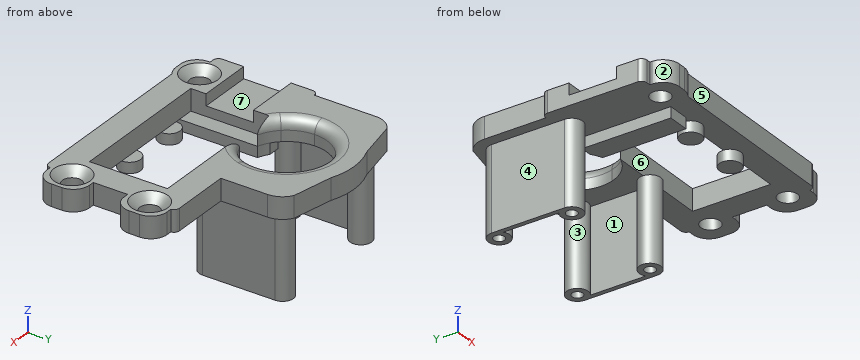
```python
from build123d import *

# Parameters (mm, degrees)
BOSS_EXTRUDE1_DEPTH                                  = 4
SKETCH5_W                                            = 5.2
SKETCH5_H                                            = 8.8
SKETCH5_W_2                                          = 5
CUT_EXTRUDE1_DEPTH                                   = 2.15
FILLET1_R                                            = 1
BOSS_EXTRUDE2_OUTLINE_R                              = 1
BOSS_EXTRUDE2_DEPTH                                  = 15.61
BOSS_EXTRUDE5_START                                  = -5
BOSS_EXTRUDE5_DEPTH                                  = 5
BOSS_EXTRUDE8_DEPTH                                  = 4
FILLET3_R                                            = 2
SKETCH9_R                                            = 2
BOSS_EXTRUDE9_DEPTH                                  = 2
SKETCH10_W                                           = 27.2
SKETCH10_H                                           = 14.5
SKETCH10_W_2                                         = 27
SKETCH10_H_2                                         = 14.3
CUT_EXTRUDE4_DEPTH                                   = 4
BOSS_EXTRUDE10_START                                 = 2
BOSS_EXTRUDE10_DEPTH                                 = 2
SKETCH12_W                                           = 8
SKETCH12_H                                           = 8
SKETCH12_W_2                                         = 6.2
SKETCH12_H_2                                         = 6.2
BOSS_EXTRUDE11_DEPTH                                 = 4
FILLET4_R                                            = 3
FILLET5_R                                            = 3
CSK_FOR_M3_HEX_SOCKET_COUNTERSUNK_CAP_SC_D           = 3.6
CSK_FOR_M3_HEX_SOCKET_COUNTERSUNK_CAP_SC_DEPTH       = 14.44
CSK_FOR_M3_HEX_SOCKET_COUNTERSUNK_CAP_SC_CSINK_D     = 6.72
CSK_FOR_M3_HEX_SOCKET_COUNTERSUNK_CAP_SC_CSINK_ANGLE = 90
CSK_FOR_M3_HEX_SOCKET_COUNTERSUNK_CAP_SC_TIP         = 1.081549114


# Read off the part's stored shape, not the designer's step: Boss-Extrude2
with BuildPart() as part:
    # Sketch3 → Boss-Extrude1 (new body)
    with BuildSketch(Plane.XY):
        with BuildLine():
            Line((5, 19.3), (-9.345122918, 19.3))
            ThreePointArc((-9.345122918, 19.3), (-23.0857932, 33.91726612), (-33.128131381, 16.55))
            Line((-33.128131381, 16.55), (-37.2, 16.55))
            Line((-37.2, 16.55), (-37.2, -2.25))
            Line((-37.2, -2.25), (-32, -2.25))
            Line((-32, -2.25), (-32, -5))
            Line((-32, -5), (5, -5))
            Line((5, -5), (5, 19.3))
        make_face()
        with BuildLine():
            ThreePointArc((-23.75, 14.3), (-25.677557149, 15.173169561), (-27.284491991, 16.55))
            ThreePointArc((-27.284491991, 16.55), (-19.55505766, 28.701473224), (-19.55, 14.3))
            Line((-19.55, 14.3), (0, 14.3))
            Line((0, 14.3), (0, 0))
            Line((0, 0), (-27, 0))
            Line((-27, 0), (-27, 14.3))
            Line((-27, 14.3), (-23.75, 14.3))
        make_face(mode=Mode.SUBTRACT)
    extrude(amount=BOSS_EXTRUDE1_DEPTH)

    # Sketch5 → Cut-Extrude1 (cut)
    with BuildSketch(Plane.XY.offset(4)):
        with Locations((-29.6, 7.15)):
            Rectangle(SKETCH5_W, SKETCH5_H)
        with Locations((-34.7, 7.15)):
            Rectangle(SKETCH5_W_2, SKETCH5_H)
    extrude(amount=-CUT_EXTRUDE1_DEPTH, mode=Mode.SUBTRACT)

    # Fillet1
    fillet1_edges = [part.edges().sort_by_distance(p)[0] for p in [
        (5, 19.3, 2),
        (5, -5, 2),
        (-32, -5, 2),
        (-32, -2.25, 2),
        (-37.2, -2.25, 2),
        (-37.2, 16.55, 2),
    ]]
    fillet(fillet1_edges, radius=FILLET1_R)

    # Boss-Extrude2 outline → Boss-Extrude2 (add)
    # profile 1 of 2: a face of its own
    with BuildSketch(Plane.XY.offset(-15.61)):
        with BuildLine():
            ThreePointArc((-9.15, 28), (-12.938854382, 28.894427191), (-9.95, 26.4))
            Line((-9.95, 26.4), (-9.95, 16.1))
            ThreePointArc((-9.95, 16.1), (-12.938854382, 13.605572809), (-9.15, 14.5))
            Line((-9.15, 14.5), (-9.15, 28))
        make_face()
        with Locations((-11.15, 14.5)):
            Circle(BOSS_EXTRUDE2_OUTLINE_R, mode=Mode.SUBTRACT)
        with Locations((-11.15, 28)):
            Circle(BOSS_EXTRUDE2_OUTLINE_R, mode=Mode.SUBTRACT)
    # profile 2 of 2: a face of its own
    with BuildSketch(Plane.XY.offset(-15.61)):
        with BuildLine():
            ThreePointArc((-33.35, 26.4), (-30.361145618, 28.894427191), (-34.15, 28))
            Line((-34.15, 28), (-34.15, 14.5))
            ThreePointArc((-34.15, 14.5), (-30.361145618, 13.605572809), (-33.35, 16.1))
            Line((-33.35, 16.1), (-33.35, 26.4))
        make_face()
        with Locations((-32.15, 14.5)):
            Circle(BOSS_EXTRUDE2_OUTLINE_R, mode=Mode.SUBTRACT)
        with Locations((-32.15, 28)):
            Circle(BOSS_EXTRUDE2_OUTLINE_R, mode=Mode.SUBTRACT)
    extrude(amount=BOSS_EXTRUDE2_DEPTH)

    # Sketch7 → Boss-Extrude5 (add)
    with BuildSketch(Plane.XY.offset(BOSS_EXTRUDE5_START)):
        with BuildLine():
            Line((-13.139974874, 14.3), (-11.15, 15.313011827))
            Line((-11.15, 15.313011827), (-9.160025126, 14.3))
            ThreePointArc((-9.160025126, 14.3), (-11.15, 12.5), (-13.139974874, 14.3))
        make_face()
    extrude(amount=BOSS_EXTRUDE5_DEPTH)

    # Sketch8 → Boss-Extrude8 (add)
    with BuildSketch(Plane(origin=(0, 0, 0), x_dir=(-1, 0, 0), z_dir=(0, 0, -1))):
        with BuildLine():
            ThreePointArc((12.211302304, 29.695180645), (14.32299851, 31.627440405), (16.818882283, 33.02867302))
            Line((16.818882283, 33.02867302), (9.212271747, 31.499315535))
            ThreePointArc((9.212271747, 31.499315535), (7.703921576, 30.030897214), (7.15, 28))
            Line((7.15, 28), (7.15, 21.5))
            Line((7.15, 21.5), (7.15, 19.3))
            Line((7.15, 19.3), (9.15, 19.3))
            Line((9.15, 19.3), (9.15, 21.5))
            Line((9.15, 21.5), (9.15, 28))
            ThreePointArc((9.15, 28), (10.181135873, 29.749657768), (12.211302304, 29.695180645))
        make_face()
        with BuildLine():
            Line((9.15, 19.3), (9.95, 19.3))
            Line((9.95, 19.3), (9.95, 25.9))
            ThreePointArc((9.95, 25.9), (10.02628451, 26.097742729), (10.105910811, 26.294163617))
            ThreePointArc((10.105910811, 26.294163617), (12.850530293, 26.947290771), (12.211302304, 29.695180645))
            ThreePointArc((12.211302304, 29.695180645), (10.181135873, 29.749657768), (9.15, 28))
            Line((9.15, 28), (9.15, 21.5))
            Line((9.15, 21.5), (9.15, 19.3))
        make_face()
        with BuildLine():
            Line((34.15, 28), (34.15, 21.5))
            Line((34.15, 21.5), (34.15, 16.55))
            Line((34.15, 16.55), (36.15, 16.55))
            Line((36.15, 16.55), (36.15, 21.5))
            Line((36.15, 21.5), (36.15, 28))
            ThreePointArc((36.15, 28), (35.596078424, 30.030897214), (34.087728253, 31.499315535))
            Line((34.087728253, 31.499315535), (26.481117717, 33.02867302))
            ThreePointArc((26.481117717, 33.02867302), (28.97700149, 31.627440405), (31.088697696, 29.695180645))
            ThreePointArc((31.088697696, 29.695180645), (33.118864127, 29.749657768), (34.15, 28))
        make_face()
        with BuildLine():
            Line((33.35, 21.5), (34.15, 21.5))
            Line((34.15, 21.5), (34.15, 28))
            ThreePointArc((34.15, 28), (33.118864127, 29.749657768), (31.088697696, 29.695180645))
            ThreePointArc((31.088697696, 29.695180645), (30.449469707, 26.947290771), (33.194089189, 26.294163617))
            ThreePointArc((33.194089189, 26.294163617), (33.27371549, 26.097742729), (33.35, 25.9))
            Line((33.35, 25.9), (33.35, 21.5))
        make_face()
        with BuildLine():
            Line((34.15, 16.55), (34.15, 21.5))
            Line((34.15, 21.5), (33.35, 21.5))
            Line((33.35, 21.5), (33.35, 17.1))
            ThreePointArc((33.35, 17.1), (33.242328005, 16.82368399), (33.128131381, 16.55))
            Line((33.128131381, 16.55), (33.35, 16.55))
            Line((33.35, 16.55), (33.35, 16.1))
            ThreePointArc((33.35, 16.1), (30.361145618, 13.605572809), (34.15, 14.5))
            Line((34.15, 14.5), (34.15, 16.55))
        make_face()
        with BuildLine():
            Line((29.15, 21.5), (33.35, 21.5))
            Line((33.35, 21.5), (33.35, 25.9))
            ThreePointArc((33.35, 25.9), (33.27371549, 26.097742729), (33.194089189, 26.294163617))
            ThreePointArc((33.194089189, 26.294163617), (30.449469707, 26.947290771), (31.088697696, 29.695180645))
            ThreePointArc((31.088697696, 29.695180645), (28.97700149, 31.627440405), (26.481117717, 33.02867302))
            Line((26.481117717, 33.02867302), (21.65, 34))
            Line((21.65, 34), (16.818882283, 33.02867302))
            ThreePointArc((16.818882283, 33.02867302), (14.32299851, 31.627440405), (12.211302304, 29.695180645))
            ThreePointArc((12.211302304, 29.695180645), (12.850530293, 26.947290771), (10.105910811, 26.294163617))
            ThreePointArc((10.105910811, 26.294163617), (10.02628451, 26.097742729), (9.95, 25.9))
            Line((9.95, 25.9), (9.95, 19.3))
            Line((9.95, 19.3), (14.479923292, 19.3))
            ThreePointArc((14.479923292, 19.3), (20.537699526, 28.917060581), (29.15, 21.5))
        make_face()
    extrude(amount=-BOSS_EXTRUDE8_DEPTH)

    # Fillet3
    fillet3_edges = [part.edges().sort_by_distance(p)[0] for p in [
        (-20.537699526, 28.917060581, 4),
    ]]
    fillet(fillet3_edges, radius=FILLET3_R)

    # Sketch9 → Boss-Extrude9 (add)
    with BuildSketch(Plane(origin=(0, 0, 0), x_dir=(-1, 0, 0), z_dir=(0, 0, -1))):
        with Locations((10.589759588, 0)):
            Circle(SKETCH9_R)
        with Locations((21.179764077, 0)):
            Circle(SKETCH9_R)
    extrude(amount=BOSS_EXTRUDE9_DEPTH)

    # Sketch10 → Cut-Extrude4 (cut)
    with BuildSketch(Plane.XY.offset(4)):
        with Locations((-13.5, 7.15)):
            Rectangle(SKETCH10_W, SKETCH10_H)
        with Locations((-13.5, 7.15)):
            Rectangle(SKETCH10_W_2, SKETCH10_H_2, mode=Mode.SUBTRACT)
    extrude(amount=-CUT_EXTRUDE4_DEPTH, mode=Mode.SUBTRACT)

    # Sketch11 → Boss-Extrude10 (add)
    with BuildSketch(Plane(origin=(0, 0, 0), x_dir=(-1, 0, 0), z_dir=(0, 0, -1)).offset(BOSS_EXTRUDE10_START)):
        with BuildLine():
            Line((24.066609195, -0.1), (24.066609195, 14.4))
            ThreePointArc((24.066609195, 14.4), (25.07672129, 14.828599757), (26.013484846, 15.4))
            Line((26.013484846, 15.4), (28.1, 15.4))
            Line((28.1, 15.4), (28.1, -0.1))
            Line((28.1, -0.1), (28.1, -1.1))
            Line((28.1, -1.1), (24.066609195, -1.1))
            Line((24.066609195, -1.1), (24.066609195, -0.1))
        make_face()
    extrude(amount=-BOSS_EXTRUDE10_DEPTH)

    # Sketch12 → Boss-Extrude11 (add)
    with BuildSketch(Plane.XY.offset(4)):
        with Locations((5, 0)):
            Rectangle(SKETCH12_W, SKETCH12_H)
        with Locations((5, 14.4)):
            Rectangle(SKETCH12_W, SKETCH12_H)
        with Locations((-32.292893219, -2.542893219)):
            Rectangle(SKETCH12_W_2, SKETCH12_H_2)
    extrude(amount=-BOSS_EXTRUDE11_DEPTH)

    # Fillet4
    fillet4_edges = [part.edges().sort_by_distance(p)[0] for p in [
        (9, 4, 2),
        (9, -4, 2),
        (9, 10.4, 2),
        (9, 18.4, 2),
        (-35.392893219, -5.642893219, 2),
    ]]
    fillet(fillet4_edges, radius=FILLET4_R)

    # Fillet5
    # the kernel refuses this fillet: 3 mm, written as the material it takes off along each edge
    with BuildSketch(Plane(origin=(-29.192893219, -5.642893219, 8.63953636), x_dir=(-1, 0, 0), z_dir=(0, 0, -1))) as fillet5_piece_1:
        with BuildLine():
            CenterArc((1.855814544, 3), FILLET5_R, 231.785675488, 38.214324512)
            Line((0, 0.642893219), (-0.037116291, 0.595751083))
            ThreePointArc((-0.037116291, 0.595751083), (-0.06, 0.321446609), (-0.06, 0))
            Line((-0.06, 0), (0, -0.06))
            Line((0, -0.06), (1.855814544, -0.06))
            Line((1.855814544, -0.06), (1.855814544, 0))
        make_face()
    extrude(amount=13.27907272, mode=Mode.SUBTRACT)

    # CSK for M3 Hex Socket Countersunk Cap Screw1
    with Locations(Plane.XY.offset(4)):
        with Locations((4.900331387, 0), (4.900331387, 14.4), (-31.553809286, -1.547116477)):
            CounterSinkHole(CSK_FOR_M3_HEX_SOCKET_COUNTERSUNK_CAP_SC_D / 2, CSK_FOR_M3_HEX_SOCKET_COUNTERSUNK_CAP_SC_CSINK_D / 2, depth=CSK_FOR_M3_HEX_SOCKET_COUNTERSUNK_CAP_SC_DEPTH, counter_sink_angle=CSK_FOR_M3_HEX_SOCKET_COUNTERSUNK_CAP_SC_CSINK_ANGLE)
            with Locations((0, 0, -(CSK_FOR_M3_HEX_SOCKET_COUNTERSUNK_CAP_SC_DEPTH + CSK_FOR_M3_HEX_SOCKET_COUNTERSUNK_CAP_SC_TIP / 2))):  # 118° drill point
                Cone(0, CSK_FOR_M3_HEX_SOCKET_COUNTERSUNK_CAP_SC_D / 2, CSK_FOR_M3_HEX_SOCKET_COUNTERSUNK_CAP_SC_TIP, mode=Mode.SUBTRACT)


solid = part.part
```
Work out the finished part from the listing and answer in its coordinate system (mm). Face numbers are marked on the shaded views. A direction names the side the tool comes from. Round coordinates to 2 decimals unless told otherwise and drop trailing zeros. Loops run counter-clockwise (first coordinate to the right, second up) from the corner with the lowest first, then second, coordinate; pieces in that order, holes last. Notation, with made-up numbers: (4.25, 68.5) -> (14.25, 68.5) arc R24 cw to (14.25, 94.5) -> close; hole circle Ø8 at (44, 44). An arc over 180 degrees is marked (long way). Write each question's results on one line, items separated by ' | '. Start each with the question number.
1. For a pull along Y with two mould halves and no side action, classify the marked faces 1, 2, 3 and 4 as +Y half, -Y half, draft (parallel to the pull), parting line (faces both ways), or undercut.
2. Section A-A (z = -7.5) is taken. Determine the outline of the cut face in (x, y).
3. A tool of negligible diameter and unlimited length cuts with its end or side. For the marked faces 5, 6 and 7, from which of +Z, -Z, +X, -X, +Y, -Y can it reach the whole face along a straight path? Write none if from no direction.
4. Given pin 1 Ø2 at (x, z) = (-32.5, -5.5) entering from +Y; pin 2 Ø2 at (y, z) = (15, -12) entering from -X; pin 3 Ø1.1 at (x, z) = (-31, 3) entering from +Y; pin 4 Ø3 at (x, y) = (-31.55, -1.55) entering from -Z, each flat-ended and moving along its own axis, determine where each tip first touches the part or whether it passes through.
5. Section B-B (y = 8) is taken. Determine the outline of the cut face in (x, z).
6. Find the intervals of material crossed by probe 1 along X at (y, z) = (21.5, 1.3); probe 2 along X at (y, z) = (0, 0.9); probe 3 along X at (y, z) = (18, -12.5), in increasing order. Write a range as from..to.
Evaluation:
1) face 1: undercut | face 2: -Y half | face 3: undercut | face 4: draft
2) outline: (-34.15, 14.5) arc R2 ccw (long way) to (-33.35, 16.1) -> (-33.35, 26.4) arc R2 ccw (long way) to (-34.15, 28) -> close; (-9.95, 16.1) arc R2 ccw (long way) to (-9.15, 14.5) -> (-9.15, 28) arc R2 ccw (long way) to (-9.95, 26.4) -> close; hole circle Ø2 at (-32.15, 14.5); hole circle Ø2 at (-32.15, 28); hole circle Ø2 at (-11.15, 14.5); hole circle Ø2 at (-11.15, 28)
3) face 5: +Z, -Z, +X, -Y | face 6: +Z | face 7: +Z, -X
4) pin 1: stops at y = 30 | pin 2: stops at x = -34.15 | pin 3: stops at y = 32.23 | pin 4: passes through
5) outline: (-37.2, 0) -> (-28.1, 0) -> (-28.1, -2) -> (-24.07, -2) -> (-24.07, 0) -> (-27.1, 0) -> (-27.1, 1.85) -> (-37.2, 1.85) -> close; (0.1, 0) -> (5, 0) -> (5, 4) -> (0.1, 4) -> close
6) probe 1: x = -36.15..-29.15, -14.15..-7.15 | probe 2: x = -37.2..-32.47, -30.63..-27.1, 0.1..3.1, 6.7..9 | probe 3: x = -34.15..-33.35, -9.95..-9.15
